Source: three-view drawing plus pictorial views. Frame: mm from the lowest corner of the part. A direction names the side the tool comes from. Give positions to 0.01 mm unless a question says otherwise; leave off trailing zeros. Order: outer loops, then holes, each group sorted by start corner. A loop starts at its lowest first (then second) coordinate and runs counter-clockwise, first axis right, second up. Notation, with made-up numbers: M 1.5,18 L 26.5,18 A26 cw 26.5,48 Z; hole C 48,41.25 d3. An arc over 180 degrees is marked long. Use CSV: the item, a comma, the result in double quotes.
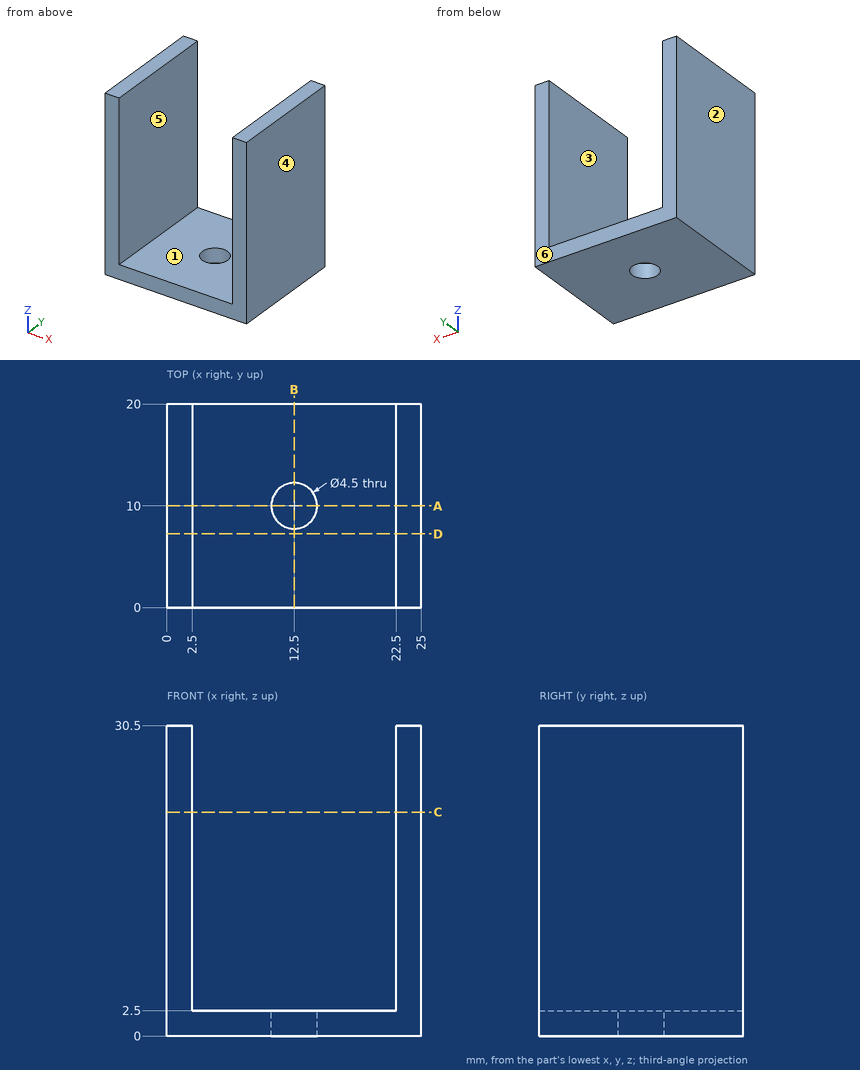
1. Pin query (flat end, axial travel): pin 1 Ø4 at (x, y) = (10.5, 7.5) entering from +Z. Return the tip coordinate at first contact, or that it passes through.
Answer:
pin 1,"z = 2.5"
2. Line query: line 1 (X direction, y = 14.75, z = 15.5); line 2 (Y direction, x = 12.5, z = 1.1); line 3 (Z direction, x = 13, y = 4.5). Output: solid intervals per line, ascending.
Answer:
line 1,"0 to 2.5, 22.5 to 25"
line 2,"0 to 7.75, 12.25 to 20"
line 3,"0 to 2.5"
3. Section D-D, the plane y = 7.25. Return the cut outline in (x, z), plus the area to 4 significant figures.
Answer:
outline,"M 0,0 L 25,0 L 25,30.5 L 22.5,30.5 L 22.5,2.5 L 2.5,2.5 L 2.5,30.5 L 0,30.5 Z"
area,"202.5 mm2"
4. Section A-A, the plane y = 10. Return the cut outline in (x, z).
Answer:
outline,"M 0,0 L 10.25,0 L 10.25,2.5 L 2.5,2.5 L 2.5,30.5 L 0,30.5 Z; M 14.75,0 L 25,0 L 25,30.5 L 22.5,30.5 L 22.5,2.5 L 14.75,2.5 Z"
5. Section B-B, the plane x = 12.5. Return the cut outline in (y, z).
Answer:
outline,"M 0,0 L 7.75,0 L 7.75,2.5 L 0,2.5 Z; M 12.25,0 L 20,0 L 20,2.5 L 12.25,2.5 Z"
6. Pull-direction query (X, two-part tool) for the marked faces 3, 4, 5 and 6; classes: +X half, -X half, draft (parallel to the pull), parting line (faces both ways), or undercut.
Answer:
face 3,"undercut"
face 4,"+X half"
face 5,"undercut"
face 6,"draft"
7. Reachability of the marked faces 1 and 2 from +Z, -Z, +X, -X, +Y, -Y: full face, straight path, thin tool, end or side. Return the list, or none.
Answer:
face 1,"+Z, +Y, -Y"
face 2,"+Z, -Z, -X, +Y, -Y"
8. Section C-C, the plane z = 22. Return the cut outline in (x, y).
Answer:
outline,"M 0,0 L 2.5,0 L 2.5,20 L 0,20 Z; M 22.5,0 L 25,0 L 25,20 L 22.5,20 Z"
